Can you work these out from the model? Positions are in its coordinate system, mm. A direction names the side the tool comes from. Round coordinates to 2 decimals unless told otherwise and drop trailing zeros. Write each loop counter-clockwise with the first axis right and the second up, starting at its lowest first coordinate (ties: lowest second). Pieces come first, ordered by that corner, then holes. Notation, with made-up numbers: M 27.25,13.25 L 40.25,13.25 A25 cw 40.25,26.25 Z; hole C 49.5,-25 d3. An arc over 180 degrees is marked long. Answer in a Markdown table with one row per item. Add a question column.
(1) I'm going to push flat-ended pins straight in: pin 1 (2 mm diameter, centred on x = -11, z = 13, fed in from +Y); pin 2 (2 mm diameter, centred on x = -12.5, z = -12.5, fed in from -Y); pin 3 (2.5 mm diameter, centred on x = 4, y = -3, fed in from -Z); pin 4 (1.4 mm diameter, centred on y = 3, z = 2, fed in from +X). Where does each tip first touch, or does it pass through?
(2) Suppose I cut it at B-B, the plane y = 0. Write out the boundary of the cut face in (x, z).
(3) If I drill on probe 1 along Z at (x, y) = (-12.5, -0.45); probe 2 along X at (y, z) = (3.25, -8.5); probe 3 along Y at (x, z) = (-11, 11.5), over which ranges is the centre line in solid material (lowest first)?
(4) If we mould it in two halves opening along X, with no side actions, what happens to faces 4 (the face through (-13.054, -0.014, 13.565)), 5 (the face through (0, 1, -12)), 6 (the face through (-17.1, 0, 0))? For each: released by +X, released by -X, zero draft, split by the parting line, or undercut.
(5) Suppose I cut it at D-D, the plane z = -7.5. Write out the boundary of the cut face in (x, y), then the cut area to 3 significant figures.
(6) Suppose I cut it at C-C, the plane x = 12. Write out the boundary of the cut face in (y, z), then the cut area to 3 significant figures.
(7) For faces 1 (the face through (10, -2, 0)), 2 (the face through (-10, 2, 0)), 3 (the face through (0, -2, 10)), which set-ups out of +Z, -Z, +X, -X, +Y, -Y let a thin tool reach every point of the face, with its end or its side?
(8) Suppose I cut it at A-A, the plane z = 12.5. Write out the boundary of the cut face in (x, y), then the cut area to 3 significant figures.
from build123d import *

# Parameters (mm, degrees)
SKETCH1_W            = 34.2
SKETCH1_H            = 34.2
BOSS_EXTRUDE1_DEPTH  = 3.9
M2_CLEARANCE_HOLE1_D = 2.4
CUT_EXTRUDE1_START   = -2.9
SKETCH9_W            = 34.2
SKETCH9_H            = 34.2
SKETCH9_R            = 1.2
SKETCH9_W_2          = 20
SKETCH9_H_2          = 20
CUT_EXTRUDE1_DEPTH   = 2.9


with BuildPart() as part:
    # Sketch1 → Boss-Extrude1 (new, symmetric)
    with BuildSketch(Plane(origin=(0, 0, 0), x_dir=(1, 0, 0), z_dir=(0, 1, 0))):
        Rectangle(SKETCH1_W, SKETCH1_H)
    extrude(amount=BOSS_EXTRUDE1_DEPTH, both=True)

    # M2 Clearance Hole1 (through all)
    with Locations(Plane(origin=(0, 3.9, 0), x_dir=(1, 0, 0), z_dir=(0, 1, 0))):
        with Locations((-12.5, 12.5), (12.5, -12.5), (12.5, 12.5), (-12.5, -12.5)):
            Hole(M2_CLEARANCE_HOLE1_D / 2)

    # Sketch9 → Cut-Extrude1 (cut)
    with BuildSketch(Plane(origin=(0, 3.9, 0), x_dir=(1, 0, 0), z_dir=(0, 1, 0)).offset(CUT_EXTRUDE1_START)):
        Rectangle(SKETCH9_W, SKETCH9_H)
        with Locations(Location((12.5, -12.5, 0), (0, 0, 270))):
            Circle(SKETCH9_R, mode=Mode.SUBTRACT)
        with Locations(Location((-12.5, -12.5, 0), (0, 0, 270))):
            Circle(SKETCH9_R, mode=Mode.SUBTRACT)
        with Locations(Location((12.5, 12.5, 0), (0, 0, 270))):
            Circle(SKETCH9_R, mode=Mode.SUBTRACT)
        with Locations(Location((-12.5, 12.5, 0), (0, 0, 270))):
            Circle(SKETCH9_R, mode=Mode.SUBTRACT)
        Rectangle(SKETCH9_W_2, SKETCH9_H_2, mode=Mode.SUBTRACT)
    cut_extrude1 = extrude(amount=CUT_EXTRUDE1_DEPTH, mode=Mode.SUBTRACT)

    # Mirror1: Cut-Extrude1 across plane
    add(cut_extrude1.mirror(Plane.ZX), mode=Mode.SUBTRACT)


solid = part.part
Calculated:
| question | item | result |
|---|---|---|
| 1 | pin 1 | y = 1 |
| 1 | pin 2 | through |
| 1 | pin 3 | z = -10 |
| 1 | pin 4 | x = 10 |
| 2 | outline | M -17.1,-17.1 L 17.1,-17.1 L 17.1,17.1 L -17.1,17.1 Z; hole C -12.5,-12.5 d2.4; hole C -12.5,12.5 d2.4; hole C 12.5,-12.5 d2.4; hole C 12.5,12.5 d2.4 |
| 3 | probe 1 | -17.1 to -13.7, -11.3 to 11.3, 13.7 to 17.1 |
| 3 | probe 2 | -10 to 10 |
| 3 | probe 3 | -1 to 1 |
| 4 | face 4 | undercut |
| 4 | face 5 | zero draft |
| 4 | face 6 | released by -X |
| 5 | outline | M -17.1,-1 L -10,-1 L -10,-3.9 L 10,-3.9 L 10,-1 L 17.1,-1 L 17.1,1 L 10,1 L 10,3.9 L -10,3.9 L -10,1 L -17.1,1 Z |
| 5 | area | 184 mm² |
| 6 | outline | M -1,-17.1 L 1,-17.1 L 1,-13.59 L -1,-13.59 Z; M -1,-11.41 L 1,-11.41 L 1,11.41 L -1,11.41 Z; M -1,13.59 L 1,13.59 L 1,17.1 L -1,17.1 Z |
| 6 | area | 59.7 mm² |
| 7 | face 1 | +Z, -Z, +X, -Y |
| 7 | face 2 | +Z, -Z, -X, +Y |
| 7 | face 3 | +Z, +X, -X, -Y |
| 8 | outline | M -17.1,-1 L -13.7,-1 L -13.7,1 L -17.1,1 Z; M -11.3,-1 L 11.3,-1 L 11.3,1 L -11.3,1 Z; M 13.7,-1 L 17.1,-1 L 17.1,1 L 13.7,1 Z |
| 8 | area | 58.8 mm² |
